Input: part model. Units: mm. Frame: model coordinates. Face numbers are marked on the shaded views. A direction names the side the tool comes from. Round coordinates to 2 decimals unless told otherwise and drop trailing zeros. Loops run counter-clockwise (first coordinate to the right, second up) from the corner with the lowest first, then second, coordinate; pieces in that order, holes last.
(1) First-contact query: pin 1 Ø0.9 at (y, z) = (1.5, 0) entering from +X; pin 2 Ø2 at (x, z) = (6, 0) entering from +Y; pin 3 Ø0.9 at (x, y) = (2, 1.5) entering from +Z. Flat tips, straight axial feed; report the tip coordinate or a pass-through.
(2) Access query for the marked faces 1, 2 and 3. Directions: +Z, -Z, +X, -X, +Y, -Y. A direction counts if a zero-diameter tool reaches every point of the face in a straight line with its end or side. Return the directions, or none.
(3) Cut plane A-A, the plane y = 1.6. Output: boundary loops of the cut face in (x, z) (3 decimals).
(4) Cut plane D-D, the plane y = 0.8. Output: boundary loops of the cut face in (x, z).
(5) Cut plane B-B, the plane x = 7. Output: boundary loops of the cut face in (y, z).
(6) Cut plane C-C, the plane z = 0.25. Output: boundary loops of the cut face in (x, y).
(7) Line query: line 1 (X direction, y = 0.25, z = -4); line 2 (Y direction, x = -4.5, z = 0); line 3 (Y direction, x = -7, z = -0.5). Output: solid intervals per line, ascending.
(8) Draft query along X for the marked faces 4 and 5. Return one class per face: released by +X, released by -X, zero draft, split by the parting line, or undercut.
from build123d import *

# Parameters (mm, degrees)
SKETCH_1_W          = 19.6
SKETCH_1_H          = 9
EXTRUDE_1_DEPTH     = 1
CUT_EXTRUDE_1_DEPTH = 11.830050785
SKETCH_4_W          = 2.6
SKETCH_4_H          = 1.65
SKETCH_4_H_2        = 3.3
EXTRUDE_2_DEPTH     = 0.83
SKETCH_3_W          = 0.537571624
SKETCH_3_H          = 1.530011548
EXTRUDE_3_DEPTH     = 1


with BuildPart() as part:
    # 草图1 → 凸台-拉伸1 (new body)
    with BuildSketch(Plane(origin=(0, 0, 0), x_dir=(1, 0, 0), z_dir=(0, 1, 0))):
        Rectangle(SKETCH_1_W, SKETCH_1_H)
    extrude(amount=EXTRUDE_1_DEPTH)

    # 草图2 → 切除-拉伸1 (cut, through all)
    with BuildSketch(Plane(origin=(0, 1, 0), x_dir=(1, 0, 0), z_dir=(0, 1, 0))):
        with BuildLine():
            Line((0.75, 4.5), (-0.75, 4.5))
            Line((-0.75, 4.5), (-0.75, 3.65))
            ThreePointArc((-0.75, 3.65), (0, 4.4), (0.75, 3.65))
            Line((0.75, 3.65), (0.75, 4.5))
        make_face()
        with BuildLine():
            ThreePointArc((0.75, 3.65), (0, 4.4), (-0.75, 3.65))
            Line((-0.75, 3.65), (0.75, 3.65))
        make_face()
        with BuildLine():
            Line((0.75, 3.65), (-0.75, 3.65))
            ThreePointArc((-0.75, 3.65), (0, 2.9), (0.75, 3.65))
        make_face()
        with BuildLine():
            ThreePointArc((0.75, -3.65), (0, -2.9), (-0.75, -3.65))
            Line((-0.75, -3.65), (0.75, -3.65))
        make_face()
        with BuildLine():
            Line((0.75, -3.65), (-0.75, -3.65))
            ThreePointArc((-0.75, -3.65), (0, -4.4), (0.75, -3.65))
        make_face()
        with BuildLine():
            ThreePointArc((0.75, -3.65), (0, -4.4), (-0.75, -3.65))
            Line((-0.75, -3.65), (-0.75, -4.5))
            Line((-0.75, -4.5), (0.75, -4.5))
            Line((0.75, -4.5), (0.75, -3.65))
        make_face()
    extrude(amount=-CUT_EXTRUDE_1_DEPTH, mode=Mode.SUBTRACT)

    # 草图4 → 凸台-拉伸2 (add)
    with BuildSketch(Plane(origin=(0, 1, 0), x_dir=(1, 0, 0), z_dir=(0, 1, 0))):
        with Locations((-6.2, 0.825)):
            Rectangle(SKETCH_4_W, SKETCH_4_H)
        with Locations((-6.2, -0.825)):
            Rectangle(SKETCH_4_W, SKETCH_4_H)
        with Locations((-2.4, 0.825)):
            Rectangle(SKETCH_4_W, SKETCH_4_H)
        with Locations((-2.4, -0.825)):
            Rectangle(SKETCH_4_W, SKETCH_4_H)
        with Locations((2.4, 0)):
            Rectangle(SKETCH_4_W, SKETCH_4_H_2)
        with Locations((6.2, 0)):
            Rectangle(SKETCH_4_W, SKETCH_4_H_2)
    extrude(amount=EXTRUDE_2_DEPTH)

    # 草图3 → 凸台-拉伸3 (add)
    with BuildSketch(Plane(origin=(0, 1, 0), x_dir=(1, 0, 0), z_dir=(0, 1, 0))):
        Rectangle(SKETCH_3_W, SKETCH_3_H)
    extrude(amount=EXTRUDE_3_DEPTH)


solid = part.part
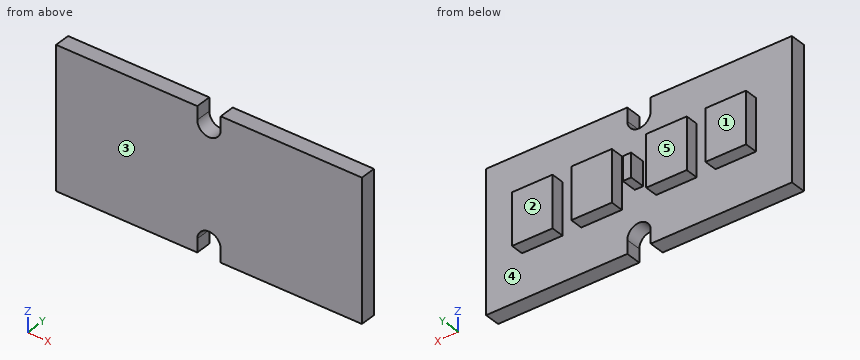
Reported:
1. pin 1: stops at x = 7.5
1. pin 2: stops at y = 1.83
1. pin 3: stops at z = 1.65
2. face 1: +Z, -Z, -X, +Y
2. face 2: +Z, -Z, +X, +Y
2. face 3: +Z, -Z, +X, -X, -Y
3. outline: (-7.5, -1.65) - (-4.9, -1.65) - (-4.9, 1.65) - (-7.5, 1.65) - close; (-3.7, -1.65) - (-1.1, -1.65) - (-1.1, 1.65) - (-3.7, 1.65) - close; (-0.269, -0.765) - (0.269, -0.765) - (0.269, 0.765) - (-0.269, 0.765) - close; (1.1, -1.65) - (3.7, -1.65) - (3.7, 1.65) - (1.1, 1.65) - close; (4.9, -1.65) - (7.5, -1.65) - (7.5, 1.65) - (4.9, 1.65) - close
4. outline: (-9.8, -4.5) - (-0.75, -4.5) - (-0.75, -3.65) arc R0.75 cw to (0.75, -3.65) - (0.75, -4.5) - (9.8, -4.5) - (9.8, 4.5) - (0.75, 4.5) - (0.75, 3.65) arc R0.75 cw to (-0.75, 3.65) - (-0.75, 4.5) - (-9.8, 4.5) - close
5. outline: (0, -4.5) - (1, -4.5) - (1, -1.65) - (1.83, -1.65) - (1.83, 1.65) - (1, 1.65) - (1, 4.5) - (0, 4.5) - close
6. outline: (-9.8, 0) - (9.8, 0) - (9.8, 1) - (7.5, 1) - (7.5, 1.83) - (4.9, 1.83) - (4.9, 1) - (3.7, 1) - (3.7, 1.83) - (1.1, 1.83) - (1.1, 1) - (0.27, 1) - (0.27, 2) - (-0.27, 2) - (-0.27, 1) - (-1.1, 1) - (-1.1, 1.83) - (-3.7, 1.83) - (-3.7, 1) - (-4.9, 1) - (-4.9, 1.83) - (-7.5, 1.83) - (-7.5, 1) - (-9.8, 1) - close
7. line 1: x = -9.8 to -0.75, 0.75 to 9.8
7. line 2: y = 0 to 1
7. line 3: y = 0 to 1.83
8. face 4: undercut
8. face 5: zero draft
